Source: CAD feature listing. Evaluate the final solid. Frame: model axes, mm. Face numbers are marked on the shaded views. A direction names the side the tool comes from. Round coordinates to 2 decimals unless told otherwise and drop trailing zeros. Write each loop counter-clockwise with the first axis right and the second up, starting at its lowest first coordinate (ties: lowest second). Pieces come first, ordered by that corner, then holes. Notation, with made-up numbers: (64.25, 65) - (110.25, 65) arc R28 cw to (110.25, 94) - close; hole circle Ø7 at (-2, -12.75). An arc over 180 degrees is marked (long way). Write item = value, one per line. Start each with the question number.
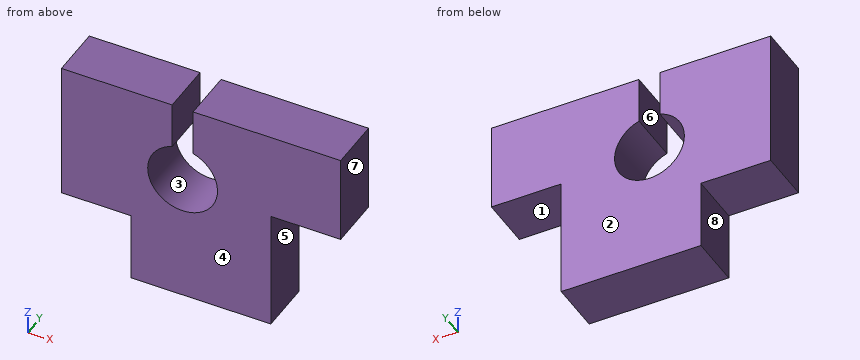
```python
from build123d import *

# Parameters (mm, degrees)
F0_W     = 101.6
F0_H     = 76.2
F1_DEPTH = 19.05
F2_W     = 25.4
F2_H     = 25.4
F3_DEPTH = 19.05
F4_W     = 25.4
F4_H     = 43.99407
F5_DEPTH = 19.05
F6_R     = 12.7
F7_DEPTH = 19.05
F8_W     = 7.62
F8_H     = 25.4
F9_DEPTH = 19.05


with BuildPart() as f1:
    # F0 (on Front) → F1 (new body)
    with BuildSketch(Plane.XZ):
        with Locations((-62.676735, -0.094059)):
            Rectangle(F0_W, F0_H)
    extrude(amount=F1_DEPTH)

    # F2 (on face) → F3 (cut)
    with BuildSketch(Plane.XZ.offset(19.05)):
        with Locations((-100.776735, -25.494059)):
            Rectangle(F2_W, F2_H)
    extrude(amount=-F3_DEPTH, mode=Mode.SUBTRACT)

    # F4 (on face) → F5 (cut)
    with BuildSketch(Plane.XZ.offset(19.05)):
        with Locations((-24.576735, -16.197024)):
            Rectangle(F4_W, F4_H)
    extrude(amount=-F5_DEPTH, mode=Mode.SUBTRACT)

    # F6 (on face) → F7 (cut)
    with BuildSketch(Plane.XZ.offset(19.05)):
        with Locations((-69.379374, 8.886294)):
            Circle(F6_R)
    extrude(amount=-F7_DEPTH, mode=Mode.SUBTRACT)

    # F8 (on face) → F9 (cut, through all)
    with BuildSketch(Plane.XZ.offset(19.05)):
        with Locations((-69.371011, 25.305941)):
            Rectangle(F8_W, F8_H)
    extrude(amount=-F9_DEPTH, mode=Mode.SUBTRACT)


solid = f1.part
```
(1) Section A-A (z = 22.5). Return the cut outline in (x, y), plus the area to 3 significant figures.
(2) Ray query, L1, parallel to X at y = -14, z = 31; L2, parallel to X at y = -9, z = 9; L3, parallel to Z at x = -92, y = -1.75. Return the intervals inside material, ascending. Write a range as from..to.
(3) Section B-B (y = -11). Return the cut outline in (x, z).
(4) Pull-direction query (Z, two-part tool) for the marked faces 1, 2 and 3; classes: +Z half, -Z half, draft (parallel to the pull), parting line (faces both ways), or undercut.
(5) Section D-D (x = -104.5). Return the cut outline in (y, z), plus the area to 3 significant figures.
(6) Reachability of the marked faces 4, 5, 6, 7 and 8 from +Z, -Z, +X, -X, +Y, -Y: full face, straight path, thin tool, end or side. Return the list, or none.
(7) Contact query for flat-ended pins moving along their axis: P1, Ø1, axis at x = -67.5, y = -16, coming from the +Z side; P2, Ø5.5, axis at y = -5, z = -21, coming from the -X side; P3, Ø5, axis at y = -11, z = -24, coming from the +X side. Output: stop coordinate, or through.
(8) Section C-C (x = -76). Return the cut outline in (y, z), plus the area to 3 significant figures.
Solution:
q1.outline = (-113.48, -19.05) - (-73.18, -19.05) - (-73.18, 0) - (-113.48, 0) - close; (-65.56, -19.05) - (-11.88, -19.05) - (-11.88, 0) - (-65.56, 0) - close
q1.area = 1,790 mm^2
q2.L1 = -113.48..-73.18, -65.56..-11.88
q2.L2 = -113.48..-82.08, -56.68..-11.88
q2.L3 = -12.79..38.01
q3.outline = (-113.48, -12.79) - (-88.08, -12.79) - (-88.08, -38.19) - (-37.28, -38.19) - (-37.28, 5.8) - (-11.88, 5.8) - (-11.88, 38.01) - (-65.56, 38.01) - (-65.56, 21) arc R12.7 cw (long way) to (-73.18, 21) - (-73.18, 38.01) - (-113.48, 38.01) - close
q4.face_1 = -Z half
q4.face_2 = draft
q4.face_3 = undercut
q5.outline = (-19.05, -12.79) - (0, -12.79) - (0, 38.01) - (-19.05, 38.01) - close
q5.area = 968 mm^2
q6.face_4 = +Z, -Z, +X, -X, -Y
q6.face_5 = -Z, +X, +Y, -Y
q6.face_6 = +Z, +Y, -Y
q6.face_7 = +Z, -Z, +X, +Y, -Y
q6.face_8 = -Z, -X, +Y, -Y
q7.P1 = -3.59
q7.P2 = -88.08
q7.P3 = -37.28
q8.outline = (-19.05, -38.19) - (0, -38.19) - (0, -1.95) - (-19.05, -1.95) - close; (-19.05, 19.72) - (0, 19.72) - (0, 38.01) - (-19.05, 38.01) - close
q8.area = 1,040 mm^2
